Source: three-view drawing plus pictorial views. Frame: mm from the lowest corner of the part. A direction names the side the tool comes from. Give positions to 0.01 mm unless a question says otherwise; leave off trailing zeros. Loops run counter-clockwise (first coordinate to the right, second up) from the corner with the lowest first, then second, coordinate; pieces in that order, holes last.
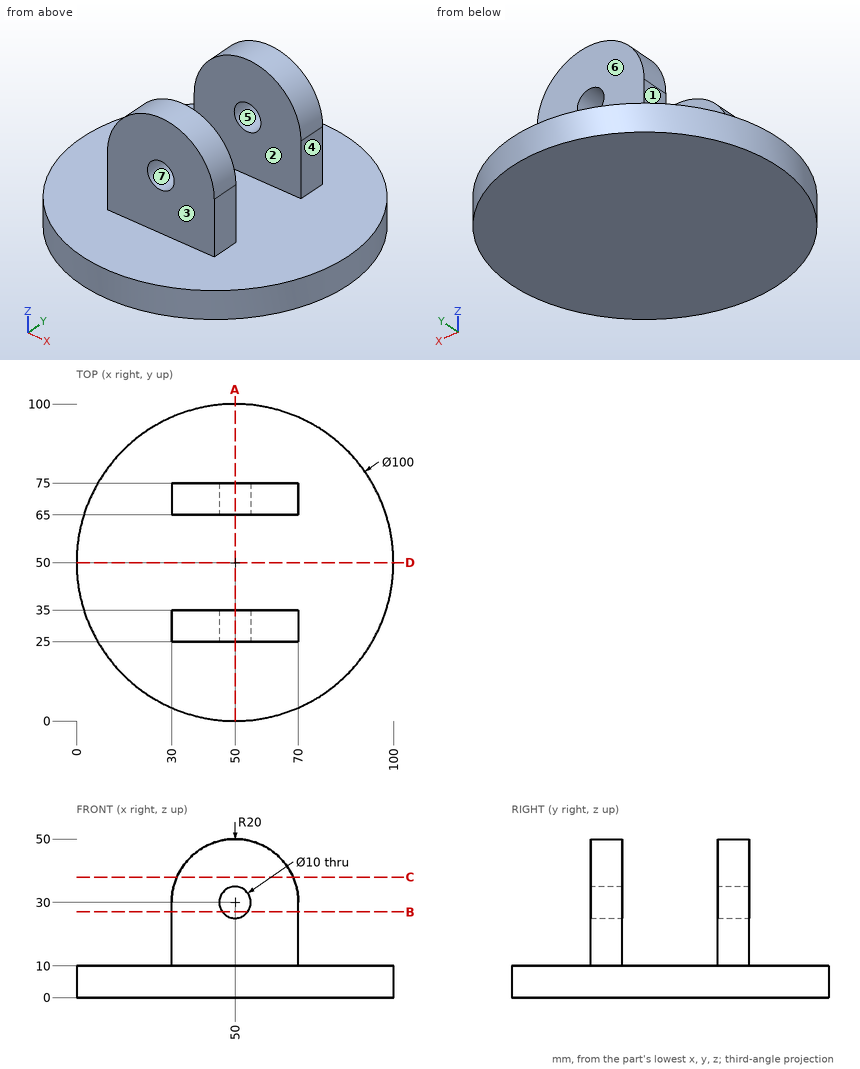
(1) Cut plane A-A (x = 50). Return the cut outline in (y, z).
Values follow:
outline: (0, 0) - (100, 0) - (100, 10) - (75, 10) - (75, 25) - (65, 25) - (65, 10) - (35, 10) - (35, 25) - (25, 25) - (25, 10) - (0, 10) - close; (25, 35) - (35, 35) - (35, 50) - (25, 50) - close; (65, 35) - (75, 35) - (75, 50) - (65, 50) - close
(2) Pin query (flat end, axial travel): pin 1 Ø13 at (x, z) = (50, 30) entering from +Y; pin 2 Ø5 at (x, y) = (54.5, 39) entering from -Z; pin 3 Ø3 at (y, z) = (28.5, 25) entering from +X; pin 4 Ø5 at (y, z) = (31, 23.5) entering from -X. Return the tip coordinate at first contact, or that it passes through.
Values follow:
pin 1: stops at y = 75
pin 2: stops at z = 0
pin 3: stops at x = 70
pin 4: stops at x = 30
(3) Ray query, probe 1 along X at (y, z) = (31, 30); probe 2 along Y at (x, z) = (58.5, 40); probe 3 along Z at (x, y) = (68, 44.5). Return the intervals inside material, ascending.
Values follow:
probe 1: x = 30 to 45, 55 to 70
probe 2: y = 25 to 35, 65 to 75
probe 3: z = 0 to 10
(4) Reachability of the marked faces 1, 2 and 3 from +Z, -Z, +X, -X, +Y, -Y: full face, straight path, thin tool, end or side. Return the list, or none.
Values follow:
face 1: +Z, -X, +Y, -Y
face 2: +Z, +X, -X
face 3: +Z, +X, -X, -Y
(5) Cut plane D-D (y = 50). Return the cut outline in (x, z).
Values follow:
outline: (0, 0) - (100, 0) - (100, 10) - (0, 10) - close
(6) Cut plane B-B (z = 27). Return the cut outline in (x, y).
Values follow:
outline: (30, 25) - (46, 25) - (46, 35) - (30, 35) - close; (30, 65) - (46, 65) - (46, 75) - (30, 75) - close; (54, 25) - (70, 25) - (70, 35) - (54, 35) - close; (54, 65) - (70, 65) - (70, 75) - (54, 75) - close
(7) Mould query, pull axis X, two halves, no side actions, for the marked faces 4, 5, 6 and 7. Classes: +X half, -X half, draft (parallel to the pull), parting line (faces both ways), or undercut.
Values follow:
face 4: +X half
face 5: undercut
face 6: draft
face 7: undercut
(8) Cut plane C-C (z = 38). Return the cut outline in (x, y), and give its area (3 significant figures).
Values follow:
outline: (31.67, 25) - (68.33, 25) - (68.33, 35) - (31.67, 35) - close; (31.67, 65) - (68.33, 65) - (68.33, 75) - (31.67, 75) - close
area: 733 mm2
